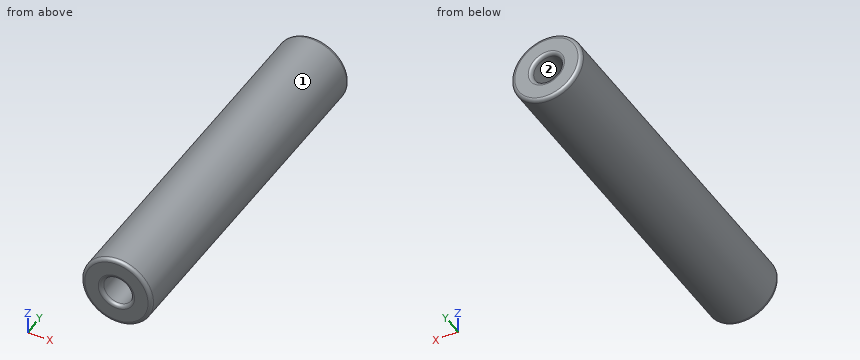
Autodesk Inventor part; units mm, degrees
ref_plane "YZ Plane" through (0, 0, 0) normal (1, 0, 0) x (0, 1, 0)
ref_plane "XZ Plane" through (0, 0, 0) normal (0, 1, 0) x (-1, 0, 0)
ref_plane "XY Plane" through (0, 0, 0) normal (0, 0, 1) x (1, 0, 0)
sketch "スケッチ1" plane through (0, 0, 0) normal (0, 1, 0) x (-1, 0, 0)
  circle A0 centre (0, 0) radius 3
  dimension "d0" = 6
extrude "押し出し1" add sketch "スケッチ1" along normal blind 30
sketch "スケッチ2" plane through (0, 30, 0) normal (0, 1, 0) x (1, 0, 0)
  circle A0 centre (0, 0) radius 1.25
  dimension "d3" = 2.5
extrude "押し出し2" cut sketch "スケッチ2" against normal blind 6
sketch "スケッチ3" plane through (0, 0, 0) normal (0, -1, 0) x (1, 0, 0)
  circle A0 centre (0, 0) radius 1.25
  circle A1 centre (0, 0) radius 1.25
  dimension "d6" = 2.5
extrude "押し出し3" cut sketch "スケッチ3" against normal blind 6
thread "ねじ1"
fillet "フィレット1" radius 0.3 4 edges at (3, 30, 0) (-1.25, 30, 0) (-1.25, 0, 0) (3, 0, 0)
properties part number "ARL-330KE"
Geometry check sheet. Reference: the model listing, model coordinates, mm. Face numbers are marked on the shaded views. Give positions to 0.01 mm unless a question says otherwise; leave off trailing zeros. Write each loop counter-clockwise with the first axis right and the second up, starting at its lowest first coordinate (ties: lowest second). Pieces come first, ordered by that corner, then holes.
1) Release check for a two-part mould opening along Z. For the marked faces 1 and 2 record: pulls with the +Z half, pulls with the -Z half, needs draft (parallel to the pull), parting line crosses it, or undercut.
2) Section check A-A, the plane x = 0. Record the boundary of the cut face in (y, z).
3) Gauge pin test, flat ends, axial feed: pin 1 (2 mm diameter, centred on y = 9.5, z = -2, fed in from +X); pin 2 (3 mm diameter, centred on x = 0, z = 0, fed in from +Y); pin 3 (2 mm diameter, centred on x = 0, z = 0, fed in from +Y). Record the tip position at first contact, or that the pin passes through.
4) Material ranges on L1, parallel to Z at x = 0, y = 2.5; L2, parallel to Y at x = -0.25, z = 0.5; L3, parallel to Z at x = 0.5, y = 24.75, recorded low to high.
5) Section check B-B, the plane z = 0. Record the boundary of the cut face in (x, y), and give its area (3 significant figures).
6) Section check C-C, the plane y = 25. Record the boundary of the cut face in (x, z), and give its area (3 significant figures).
Computed:
1. face 1: parting line crosses it
1. face 2: undercut
2. outline: (0, -2.7) arc R0.3 ccw to (0.3, -3) - (29.7, -3) arc R0.3 ccw to (30, -2.7) - (30, -1.55) arc R0.3 ccw to (29.7, -1.25) - (24, -1.25) - (24, 1.25) - (29.7, 1.25) arc R0.3 ccw to (30, 1.55) - (30, 2.7) arc R0.3 ccw to (29.7, 3) - (0.3, 3) arc R0.3 ccw to (0, 2.7) - (0, 1.55) arc R0.3 ccw to (0.3, 1.25) - (6, 1.25) - (6, -1.25) - (0.3, -1.25) arc R0.3 ccw to (0, -1.55) - close
3. pin 1: stops at x = 2.83
3. pin 2: stops at y = 30
3. pin 3: stops at y = 24
4. L1: z = -3 to -1.25, 1.25 to 3
4. L2: y = 6 to 24
4. L3: z = -2.96 to -1.15, 1.15 to 2.96
5. outline: (-3, 0.3) arc R0.3 ccw to (-2.7, 0) - (-1.55, 0) arc R0.3 ccw to (-1.25, 0.3) - (-1.25, 6) - (1.25, 6) - (1.25, 0.3) arc R0.3 ccw to (1.55, 0) - (2.7, 0) arc R0.3 ccw to (3, 0.3) - (3, 29.7) arc R0.3 ccw to (2.7, 30) - (1.55, 30) arc R0.3 ccw to (1.25, 29.7) - (1.25, 24) - (-1.25, 24) - (-1.25, 29.7) arc R0.3 ccw to (-1.55, 30) - (-2.7, 30) arc R0.3 ccw to (-3, 29.7) - close
5. area: 150 mm2
6. outline: circle Ø6 at (0, 0); hole circle Ø2.5 at (0, 0)
6. area: 23.4 mm2
